from build123d import *

# Parameters (mm, degrees)
BOSS_EXTRUDE1_DEPTH = 254
SKETCH3_R           = 2.0193
CUT_EXTRUDE1_DEPTH  = 257.615737404


with BuildPart() as part:
    # Sketch6 → Boss-Extrude1 (new body)
    with BuildSketch(Plane(origin=(0, 0, 0), x_dir=(0, 0, -1), z_dir=(1, 0, 0))):
        with BuildLine():
            Line((17.0434, 0), (32.9184, 0))
            Line((32.9184, 0), (32.9184, 15.875))
            Line((32.9184, 15.875), (31.8516, 15.875))
            ThreePointArc((31.8516, 15.875), (31.492389755, 15.726210245), (31.3436, 15.367))
            Line((31.3436, 15.367), (31.3436, 2.5908))
            ThreePointArc((31.3436, 2.5908), (31.04602049, 1.87237951), (30.3276, 1.5748))
            Line((30.3276, 1.5748), (17.5514, 1.5748))
            ThreePointArc((17.5514, 1.5748), (17.192189755, 1.426010245), (17.0434, 1.0668))
            Line((17.0434, 1.0668), (17.0434, 0))
        make_face()
    extrude(amount=-BOSS_EXTRUDE1_DEPTH)

    # Sketch3 → Cut-Extrude1 (cut, through all)
    with BuildSketch(Plane(origin=(0, 0, 0), x_dir=(1, 0, 0), z_dir=(0, 1, 0))):
        with Locations(Location((-12.7, 25.4, 0), (0, 0, 270))):
            Circle(SKETCH3_R)
        with Locations(Location((-88.9, 25.4, 0), (0, 0, 270))):
            Circle(SKETCH3_R)
        with Locations(Location((-165.1, 25.4, 0), (0, 0, 270))):
            Circle(SKETCH3_R)
        with Locations(Location((-241.3, 25.4, 0), (0, 0, 270))):
            Circle(SKETCH3_R)
    extrude(amount=CUT_EXTRUDE1_DEPTH, mode=Mode.SUBTRACT)


solid = part.part
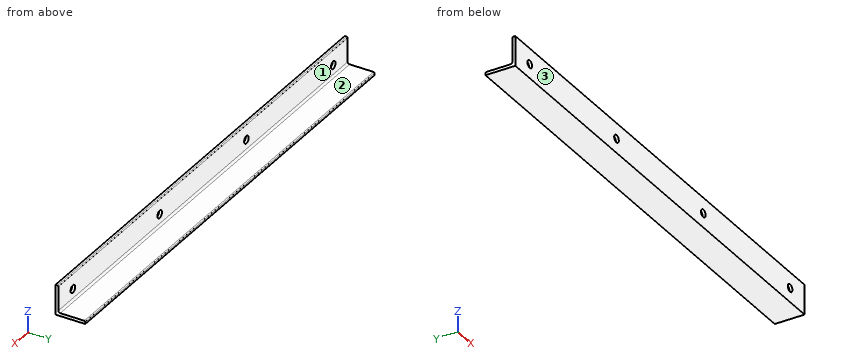
Geometry check sheet. Reference: the model listing, model coordinates, mm. Face numbers are marked on the shaded views. Give positions to 0.01 mm unless a question says otherwise; leave off trailing zeros. Order: outer loops, then holes, each group sorted by start corner. A loop starts at its lowest first (then second) coordinate and runs counter-clockwise, first axis right, second up.
1. Sectioned sample at A-A (x = -138). Record the boundary of the cut face in (y, z) (3 decimals), then the cut area to 3 significant figures.
Completed:
outline: (0, -32.918) - (15.875, -32.918) - (15.875, -31.852) arc R0.508 ccw to (15.367, -31.344) - (2.591, -31.344) arc R1.016 cw to (1.575, -30.328) - (1.575, -17.551) arc R0.508 ccw to (1.067, -17.043) - (0, -17.043) - close
area: 47.6 mm2
2. Sectioned sample at B-B (y = 6.75). Record the boundary of the cut face in (x, z), then the cut area to 3 significant figures.
Completed:
outline: (-254, -32.92) - (0, -32.92) - (0, -31.34) - (-254, -31.34) - close
area: 400 mm2
3. Draft check along Y on the marked faces 1, 2 and 3. Enter one of: pulls with the +Y half, pulls with the -Y half, needs draft (parallel to the pull), parting line crosses it, or undercut.
Completed:
face 1: pulls with the +Y half
face 2: needs draft
face 3: pulls with the -Y half
4. Depth check by flat-ended pin: pin 1 (6 mm diameter, centred on x = -205.5, z = -21.5, fed in from +Y); pin 2 (4 mm diameter, centred on x = -174, z = -29.5, fed in from +Y). Enter the tip coordinate at first touch or a pass-through.
Completed:
pin 1: stops at y = 1.57
pin 2: stops at y = 15.73
5. Scan lines: line 1 (X direction, y = 0.8, z = -25.4); line 2 (Z direction, x = -12.7, y = 0.6); line 3 (Z direction, x = -165.1, y = 1.2). Record each from-to range of solid material in increasing order.
Completed:
line 1: x = -254 to -243.32, -239.28 to -167.12, -163.08 to -90.92, -86.88 to -14.72, -10.68 to 0
line 2: z = -32.92 to -27.42, -23.38 to -17.04
line 3: z = -32.92 to -27.42, -23.38 to -17.06
